from build123d import *

# Parameters (mm, degrees)
SKETCH_R      = 9.85
SKETCH_R_2    = 3.25
PAD_DEPTH     = 10
SKETCH001_R   = 9.85
SKETCH001_R_2 = 8.15
PAD001_DEPTH  = 5.8
POCKET_DEPTH  = 6
CHAMFER_SIZE  = 1


with BuildPart() as part:
    # Sketch → Pad (new body)
    with BuildSketch(Plane.XY):
        Circle(SKETCH_R)
        Circle(SKETCH_R_2, mode=Mode.SUBTRACT)
    extrude(amount=PAD_DEPTH)

    # Sketch001 (on Face3 of Pad) → Pad001 (join)
    with BuildSketch(Plane(origin=(0, 0, 0), x_dir=(1, 0, 0), z_dir=(0, 0, -1))):
        Circle(SKETCH001_R)
        Circle(SKETCH001_R_2, mode=Mode.SUBTRACT)
    extrude(amount=PAD001_DEPTH)

    # Sketch002 (on Face3 of Pad001) → Pocket (cut)
    with BuildSketch(Plane.XY.offset(10)):
        Polygon((6.581793, 0), (3.290897, 5.7), (-3.290897, 5.7), (-6.581793, 0), (-3.290897, -5.7), (3.290897, -5.7), align=None)
    extrude(amount=-POCKET_DEPTH, mode=Mode.SUBTRACT)

    # Chamfer
    chamfer_edges = [part.edges().sort_by_distance(p)[0] for p in [
        (-9.85, 0, 10),
    ]]
    chamfer(chamfer_edges, length=CHAMFER_SIZE)


solid = part.part
Geometry check sheet. Reference: the model listing, model coordinates, mm. A direction names the side the tool comes from. Give positions to 0.01 mm unless a question says otherwise; leave off trailing zeros. Order: outer loops, then holes, each group sorted by start corner. A loop starts at its lowest first (then second) coordinate and runs counter-clockwise, first axis right, second up. Notation, with made-up numbers: (13.25, 50.5) - (17.25, 50.5) arc R13 ccw to (17.25, 59.5) - close; hole circle Ø1 at (73, 58). An arc over 180 degrees is marked (long way). Use one line per item in the form item = value.
1) Depth check by flat-ended pin: pin 1 Ø5 at (x, z) = (5, 6) entering from +Y; pin 2 Ø5 at (x, y) = (1.5, 2) entering from -Z; pin 3 Ø6 at (x, z) = (7, 1.5) entering from -Y. Enter the tip coordinate at first touch or a pass-through.
Working result:
pin_1 = 9.53
pin_2 = 0
pin_3 = -9
2) Access from +Z, -Z, +X, -X, +Y, -Y to the whole of each face (thin tool, end or side, straight path). Record for faces 1 (the face through (0, -6, 10)), 2 (the face through (-6.468, 4.959, -2.859)), 3 (the face through (0, 5.7, 7)).
Working result:
face_1 = +Z, +X, -X, +Y, -Y
face_2 = -Z
face_3 = +Z
3) Sectioned sample at B-B (z = 5.75). Record the boundary of the cut face in (x, y), and give its area (3 significant figures).
Working result:
outline = circle Ø19.7 at (0, 0); hole (-6.58, 0) - (-3.29, -5.7) - (3.29, -5.7) - (6.58, 0) - (3.29, 5.7) - (-3.29, 5.7) - close
area = 192 mm^2
4) Sectioned sample at C-C (z = -4.5). Record the boundary of the cut face in (x, y), and give its area (3 significant figures).
Working result:
outline = circle Ø19.7 at (0, 0); hole circle Ø16.3 at (0, 0)
area = 96.1 mm^2
5) Draft check along X on faces 4 (the face through (-7.82, 5.99, 1.7)), 5 (the face through (-6, -6, -5.8)), 6 (the face through (4, 0, 0)). Enter one of: released by +X, released by -X, zero draft, split by the parting line, or undercut.
Working result:
face_4 = split by the parting line
face_5 = zero draft
face_6 = undercut
6) Material ranges on probe 1 along X at (y, z) = (0, -2.75); probe 2 along X at (y, z) = (0, 2.65), recorded low to high. Write a range as from..to.
Working result:
probe_1 = -9.85..-8.15, 8.15..9.85
probe_2 = -9.85..-3.25, 3.25..9.85
7) Sectioned sample at A-A (x = 0). Record the boundary of the cut face in (y, z).
Working result:
outline = (-9.85, -5.8) - (-8.15, -5.8) - (-8.15, 0) - (-3.25, 0) - (-3.25, 4) - (-5.7, 4) - (-5.7, 10) - (-8.85, 10) - (-9.85, 9) - close; (3.25, 0) - (8.15, 0) - (8.15, -5.8) - (9.85, -5.8) - (9.85, 9) - (8.85, 10) - (5.7, 10) - (5.7, 4) - (3.25, 4) - close
8) Sectioned sample at D-D (z = 0.75). Record the boundary of the cut face in (x, y), and give its area (3 significant figures).
Working result:
outline = circle Ø19.7 at (0, 0); hole circle Ø6.5 at (0, 0)
area = 272 mm^2
